Design review of the part built by this model. Coordinates are the model's own, in mm. A direction names the side the tool comes from. Round coordinates to 2 decimals unless told otherwise and drop trailing zeros. Order: outer loops, then holes, each group sorted by start corner. A loop starts at its lowest first (then second) coordinate and runs counter-clockwise, first axis right, second up. Notation, with made-up numbers: (69.25, -13.5) - (106.25, -13.5) arc R29 ccw to (106.25, 25.5) - close; hole circle Ø11 at (24.5, -35). An arc over 180 degrees is marked (long way). Use CSV: the item, a comma, the result in double quotes. Start each with the question number.
from build123d import *

# Parameters (mm, degrees)
SKETCH1_R           = 100
BOSS_EXTRUDE1_DEPTH = 10
SKETCH2_W           = 21.2
SKETCH2_H           = 13.7
SKETCH2_W_2         = 13.7
SKETCH2_H_2         = 21.2
BOSS_EXTRUDE2_DEPTH = 30
SKETCH3_R           = 3.025
CUT_EXTRUDE1_DEPTH  = 190
SKETCH4_R           = 3.025
CUT_EXTRUDE2_DEPTH  = 190
SKETCH5_R           = 12.5
BOSS_EXTRUDE3_DEPTH = 30
CHAMFER1_SIZE       = 2


with BuildPart() as part:
    # Sketch1 → Boss-Extrude1 (new body)
    with BuildSketch(Plane(origin=(0, 0, 0), x_dir=(1, 0, 0), z_dir=(0, 1, 0))):
        with Locations(Location((0, 0, 0), (0, 0, 270))):
            Circle(SKETCH1_R)
    extrude(amount=BOSS_EXTRUDE1_DEPTH)

    # Sketch2 → Boss-Extrude2 (add)
    with BuildSketch(Plane(origin=(0, 10, 0), x_dir=(1, 0, 0), z_dir=(0, 1, 0))):
        with Locations((0, -77.5)):
            Rectangle(SKETCH2_W, SKETCH2_H)
        with Locations((77.5, 0)):
            Rectangle(SKETCH2_W_2, SKETCH2_H_2)
        with Locations((-77.5, 0)):
            Rectangle(SKETCH2_W_2, SKETCH2_H_2)
        with Locations((0, 77.5)):
            Rectangle(SKETCH2_W, SKETCH2_H)
    extrude(amount=BOSS_EXTRUDE2_DEPTH)

    # Sketch3 → Cut-Extrude1 (cut)
    with BuildSketch(Plane.ZY.offset(84.35)):
        with Locations((0, 30)):
            Circle(SKETCH3_R)
    extrude(amount=-CUT_EXTRUDE1_DEPTH, mode=Mode.SUBTRACT)

    # Sketch4 → Cut-Extrude2 (cut)
    with BuildSketch(Plane.XY.offset(84.35)):
        with Locations((0, 30)):
            Circle(SKETCH4_R)
    extrude(amount=-CUT_EXTRUDE2_DEPTH, mode=Mode.SUBTRACT)

    # Sketch5 → Boss-Extrude3 (add)
    with BuildSketch(Plane(origin=(0, 10, 0), x_dir=(1, 0, 0), z_dir=(0, 1, 0))):
        with Locations(Location((0, 0, 0), (0, 0, 90))):
            Circle(SKETCH5_R)
    extrude(amount=BOSS_EXTRUDE3_DEPTH)

    # Chamfer1
    chamfer1_edges = [part.edges().sort_by_distance(p)[0] for p in [
        (0, 40, 12.5),
    ]]
    chamfer(chamfer1_edges, length=CHAMFER1_SIZE)


solid = part.part
Q1. For L1, parallel to Y at x = -74.75, z = 0 (3 decimals); L2, parallel to Y at x = 7, z = 26.5; L3, parallel to X at y = 19, z = 83.5, list the stretches that pass through material, from the lowest coordinate up. Write a range as [from, to].
Q2. Take a section at A-A (y = 30). Give the number of separate pieces and of enclosed holes in the cut face, plus the area to 3 significant figures.
Q3. Clearance check with flat-ended pins moving along their axes: pin 1 (17 mm diameter, centred on y = 19, z = 1, fed in from +X); pin 2 (10.5 mm diameter, centred on y = 30.5, z = -2, fed in from -X); pin 3 (11 mm diameter, centred on y = 26, z = 81, fed in from -X); pin 4 (8 mm diameter, centred on y = 14.5, z = 62, fed in from +X). State where each tip first meets the part, or that it passes through.
Q4. Take a section at D-D (x = -75.5). State the section outline as (y, z) points (3 decimals), plus the area to 3 significant figures.
Q5. Take a section at B-B (x = 0). State the section outline as (y, z) points (3 decimals), plus the area to 3 significant figures.
Q6. Take a section at C-C (z = 0). State the section outline as (x, y) points (3 decimals), plus the area to 3 significant figures.
Q7. The part is to be moulded in two halves that separate along X. For faces 1 (the flat face through (-70.65, 25, 0)), 2 (the cylindrical face through (30.04, 4.93, 95.38)), 3 (the flat face through (-78, 25, -10.6)), 4 (the cylindrical face through (1.4, 27.32, 77.6)), say which applies: +X half, -X half, draft (parallel to the pull), parting line (faces both ways), or undercut.
Q8. Tool access review of faces 5 (the flat face through (10.6, 25, -77)), 6 (the flat face through (0, 25, 70.65)), 7 (the flat face through (0, 25, 84.35)), 8 (the flat face through (-84.35, 25, 0)): name each direction out of +Z, -Z, +X, -X, +Y, -Y from which nothing blocks a thin tool from reaching the whole face with its end or side.
Findings below:
1,L1,"y = [0, 26.975], [33.025, 40]"
1,L2,"y = [0, 10]"
1,L3,"x = [-10.6, 10.6]"
2,separate pieces,"9"
2,enclosed holes,"0"
2,area,"1,320 mm^2"
3,pin 1,"stops at x = 84.35"
3,pin 2,"stops at x = -84.35"
3,pin 3,"stops at x = -10.6"
3,pin 4,"passes through"
4,outline,"(0, -65.572) - (10, -65.572) - (10, -10.6) - (40, -10.6) - (40, 10.6) - (10, 10.6) - (10, 65.572) - (0, 65.572) - close; hole circle Ø6.05 at (30, 0)"
4,area,"1,920 mm^2"
5,outline,"(0, -100) - (10, -100) - (10, -84.35) - (26.975, -84.35) - (26.975, -70.65) - (10, -70.65) - (10, -12.5) - (38, -12.5) - (40, -10.5) - (40, 10.5) - (38, 12.5) - (10, 12.5) - (10, 70.65) - (26.975, 70.65) - (26.975, 84.35) - (10, 84.35) - (10, 100) - (0, 100) - close; (33.025, -84.35) - (40, -84.35) - (40, -70.65) - (33.025, -70.65) - close; (33.025, 70.65) - (40, 70.65) - (40, 84.35) - (33.025, 84.35) - close"
5,area,"3,400 mm^2"
6,outline,"(-100, 0) - (100, 0) - (100, 10) - (84.35, 10) - (84.35, 26.975) - (70.65, 26.975) - (70.65, 10) - (12.5, 10) - (12.5, 38) - (10.5, 40) - (-10.5, 40) - (-12.5, 38) - (-12.5, 10) - (-70.65, 10) - (-70.65, 26.975) - (-84.35, 26.975) - (-84.35, 10) - (-100, 10) - close; (-84.35, 33.025) - (-70.65, 33.025) - (-70.65, 40) - (-84.35, 40) - close; (70.65, 33.025) - (84.35, 33.025) - (84.35, 40) - (70.65, 40) - close"
6,area,"3,400 mm^2"
7,face 1,"undercut"
7,face 2,"parting line"
7,face 3,"draft"
7,face 4,"undercut"
8,face 5,"-Z, +X, +Y"
8,face 6,"+X, -X, +Y"
8,face 7,"+Z, +X, -X, +Y"
8,face 8,"+Z, -Z, -X, +Y"
